```python
from build123d import *

# Parameters (mm, degrees)
SKETCH1_R           = 32
BOSS_EXTRUDE1_DEPTH = 4
SKETCH3_R           = 20
SKETCH2_R           = 32
FILLET1_R           = 1
SKETCH4_R           = 4
BOSS_EXTRUDE2_DEPTH = 1.5
FILLET2_R           = 1


with BuildPart() as part:
    # Sketch1 → Boss-Extrude1 (new body)
    with BuildSketch(Plane(origin=(0, 0, 0), x_dir=(1, 0, 0), z_dir=(0, 1, 0))):
        with Locations(Location((0, 0, 0), (0, 0, 270))):
            Circle(SKETCH1_R)
    extrude(amount=BOSS_EXTRUDE1_DEPTH)

    # Sketch3 → Loft1 section 0
    with BuildSketch(Plane(origin=(0, 8, 0), x_dir=(-1, 0, 0), z_dir=(0, 1, 0))):
        Circle(SKETCH3_R)
    # Sketch2 → Loft1 section 1
    with BuildSketch(Plane(origin=(0, 4, 0), x_dir=(1, 0, 0), z_dir=(0, 1, 0))):
        Circle(SKETCH2_R)
    loft()

    # Fillet1
    fillet1_edges = [part.edges().sort_by_distance(p)[0] for p in [
        (-22.627416998, 4, 22.627416998),
    ]]
    fillet(fillet1_edges, radius=FILLET1_R)

    # Sketch4 → Boss-Extrude2 (add)
    with BuildSketch(Plane(origin=(0, 8, 0), x_dir=(1, 0, 0), z_dir=(0, 1, 0))):
        with Locations(Location((-13.5, -4, 0), (0, 0, 270))):
            Circle(SKETCH4_R)
        with Locations(Location((13.5, -4, 0), (0, 0, 270))):
            Circle(SKETCH4_R)
    extrude(amount=BOSS_EXTRUDE2_DEPTH)

    # Fillet2
    fillet2_edges = [part.edges().sort_by_distance(p)[0] for p in [
        (-13.5, 9.5, 0),
        (13.5, 9.5, 0),
    ]]
    fillet(fillet2_edges, radius=FILLET2_R)


solid = part.part
```
Read the model definition and answer for the solid it produces. Units are mm, in the model's axes. A direction names the side the tool comes from. Round coordinates to 2 decimals unless told otherwise and drop trailing zeros. Write each loop counter-clockwise with the first axis right and the second up, starting at its lowest first coordinate (ties: lowest second). Pieces come first, ordered by that corner, then holes. Notation, with made-up numbers: (69, 60.5) -> (85, 60.5) arc R18 cw to (85, 64.5) -> close; hole circle Ø10 at (79, -21). An arc over 180 degrees is marked (long way). Answer in a Markdown table with one row per item. Add a question column.
1) Which of the six approach directions +Z, -Z, +X, -X, +Y, -Y give full straight-line access (tool end or side, diameter ignored) to faces 1 (the face through (-13, 9.5, 4)), 2 (the face through (-12.299, 8.246, 7.815))?
2) Determine the mould class of faces 3 (the face through (17.466, 8.246, 3.479)), 4 (the face through (14, 9.5, 4)), 5 (the face through (-31.24, 1.62, -6.94)) for opening direction X: pulls with the +X half, pulls with the -X half, needs draft (parallel to the pull), parting line crosses it, or undercut.
3) Given P1, Ø1, axis at x = -12.5, y = 3.5, coming from the -Z side; P2, Ø5, axis at x = -4.5, y = 5, coming from the +Z side, each flat-ended and moving along its own axis, determine where each tip first touches the part or whether it passes through.
4) Find section A-A, the plane y = 1.5. Determine the outline of the cut face in (x, z).
5) Find section B-B, the plane y = 5. Determine the outline of the cut face in (x, z).
6) Consider line 1 (Y direction, x = 3, z = 12); line 2 (X direction, y = 1.75, z = -8); line 3 (Z direction, x = 7, y = 2.75). Determine where each line is inside the solid, lowest interval first.
Findings below:
| question | item | result |
|---|---|---|
| 1 | face 1 | +Z, -Z, +X, -X, +Y |
| 1 | face 2 | +Y |
| 2 | face 3 | undercut |
| 2 | face 4 | needs draft |
| 2 | face 5 | parting line crosses it |
| 3 | P1 | z = -29.65 |
| 3 | P2 | z = 31.89 |
| 4 | outline | circle Ø64 at (0, 0) |
| 5 | outline | circle Ø58 at (0, 0) |
| 6 | line 1 | 0 to 8 |
| 6 | line 2 | -30.98 to 30.98 |
| 6 | line 3 | -31.22 to 31.22 |
